from build123d import *

# Parameters (mm, degrees)
SKETCH2_W           = 140
SKETCH2_H           = 140
BOSS_EXTRUDE1_DEPTH = 10
SKETCH3_R           = 14.3
CUT_EXTRUDE1_DEPTH  = 100.498743711
CIRPATTERN1_COUNT   = 4
SKETCH4_R           = 40.5
CUT_EXTRUDE2_DEPTH  = 100.498743711


with BuildPart() as part:
    # Sketch2 → Boss-Extrude1 (new body)
    with BuildSketch(Plane.XY):
        Rectangle(SKETCH2_W, SKETCH2_H)
    extrude(amount=BOSS_EXTRUDE1_DEPTH)

    # Sketch3 → Cut-Extrude1 (cut, through all)
    with BuildSketch(Plane.XY.offset(10)):
        with Locations((-42.915392768, 34.398678224)):
            Circle(SKETCH3_R)
    cut_extrude1 = extrude(amount=-CUT_EXTRUDE1_DEPTH, mode=Mode.SUBTRACT)

    # CirPattern1: Cut-Extrude1 ×4 about axis
    cirpattern1_axis = Axis((1.454294092, -1.165684182, 0), (0, 0, 1))
    for i in range(1, CIRPATTERN1_COUNT):
        add(cut_extrude1.rotate(cirpattern1_axis, i * 360 / CIRPATTERN1_COUNT), mode=Mode.SUBTRACT)

    # Sketch4 → Cut-Extrude2 (cut, through all)
    with BuildSketch(Plane.XY.offset(10)):
        Circle(SKETCH4_R)
    extrude(amount=-CUT_EXTRUDE2_DEPTH, mode=Mode.SUBTRACT)


solid = part.part
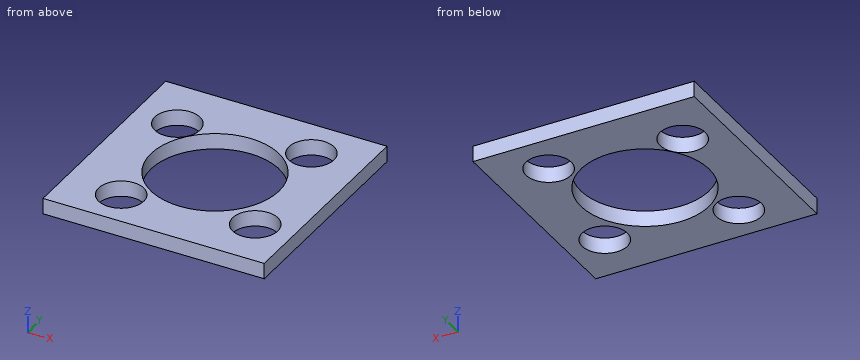
Read the model definition and answer for the solid it produces. Units are mm, in the model's axes. Give positions to 0.01 mm unless a question says otherwise; leave off trailing zeros. Write each loop counter-clockwise with the first axis right and the second up, starting at its lowest first coordinate (ties: lowest second). Pieces come first, ordered by that corner, then holes. Notation, with made-up numbers: (42.5, 50) - (99.5, 50) arc R14 cw to (99.5, 55) - close; hole circle Ø8 at (28.25, 26.25). An arc over 180 degrees is marked (long way). Return JSON: item names as keys, results as strings.
Q1. Given P1, Ø5, axis at x = 9.5, y = 36, coming from the -Z side; P2, Ø3, axis at x = 30, y = -56, coming from the -Z side, each flat-ended and moving along its own axis, determine where each tip first touches the part or whether it passes through.
Reply:
{"P1": "through", "P2": "z = 0"}
Q2. A cutting plane is placed at C-C, the plane z = 4. Determine the outline of the cut face in (x, y).
Reply:
{"outline": "(-70, -70) - (70, -70) - (70, 70) - (-70, 70) - close; hole circle Ø28.6 at (-42.92, 34.4); hole circle Ø28.6 at (-34.11, -45.54); hole circle Ø81 at (0, 0); hole circle Ø28.6 at (37.02, 43.2); hole circle Ø28.6 at (45.82, -36.73)"}
Q3. Consider line 1 along Y through (x, z) = (0, 3.75); line 2 along Y through (x, z) = (-45, 2.75); line 3 along Y through (x, z) = (-27, 4.75). Determine where each line is inside the solid, lowest interval first. Write a range as [from, to].
Reply:
{"line 1": "[-70, -40.5], [40.5, 70]", "line 2": "[-70, -54.8], [-36.27, 20.25], [48.55, 70]", "line 3": "[-70, -57.94], [-33.13, -30.19], [30.19, 70]"}
Q4. A cutting plane is placed at A-A, the plane x = 0. Determine the outline of the cut face in (y, z).
Reply:
{"outline": "(-70, 0) - (-40.5, 0) - (-40.5, 10) - (-70, 10) - close; (40.5, 0) - (70, 0) - (70, 10) - (40.5, 10) - close"}
